from build123d import *

# Parameters (mm, degrees)
F0_W     = 38.1
F0_H     = 38.1
F0_R     = 6.35
F0_R_2   = 3.175
F1_DEPTH = 25.4
F2_W     = 21.117794
F2_H     = 7.199542
F2_W_2   = 19.090971
F3_DEPTH = 38.101


with BuildPart() as f1:
    # F0 (on Top) → F1 (new body)
    with BuildSketch(Plane.XY):
        with Locations((19.05, 19.05)):
            Rectangle(F0_W, F0_H)
        with Locations((19.05, 19.05)):
            Circle(F0_R, mode=Mode.SUBTRACT)
        with BuildLine():
            Line((69.85, 38.1), (38.1, 38.1))
            Line((38.1, 38.1), (38.1, 0))
            Line((38.1, 0), (69.85, 0))
            ThreePointArc((69.85, 0), (88.9, 19.05), (69.85, 38.1))
        make_face()
        with Locations((54.437503, 8.829627)):
            Circle(F0_R_2, mode=Mode.SUBTRACT)
        with Locations((69.85, 8.829627)):
            Circle(F0_R_2, mode=Mode.SUBTRACT)
        with Locations((54.437503, 29.22605)):
            Circle(F0_R_2, mode=Mode.SUBTRACT)
        with Locations((69.85, 29.22605)):
            Circle(F0_R_2, mode=Mode.SUBTRACT)
    extrude(amount=F1_DEPTH)

    # F2 (on face) → F3 (cut, through all)
    with BuildSketch(Plane.XZ):
        with Locations((59.291103, 21.800229)):
            Rectangle(F2_W, F2_H)
        with Locations((79.395485, 21.800229)):
            Rectangle(F2_W_2, F2_H)
        with Locations((59.291103, 3.599771)):
            Rectangle(F2_W, F2_H)
        with Locations((79.395485, 3.599771)):
            Rectangle(F2_W_2, F2_H)
    extrude(amount=-F3_DEPTH, mode=Mode.SUBTRACT)


solid = f1.part
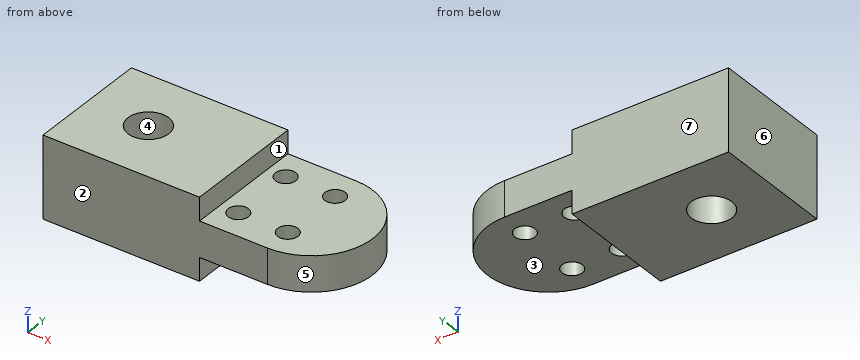
Input: part model. Units: mm. Frame: model coordinates. Face numbers are marked on the shaded views. A direction names the side the tool comes from. Round coordinates to 2 decimals unless told otherwise and drop trailing zeros. Order: outer loops, then holes, each group sorted by start corner. A loop starts at its lowest first (then second) coordinate and runs counter-clockwise, first axis right, second up.
1. Material intervals for line 1 (Y direction, x = 69.85, z = 15); line 2 (X direction, y = 31.5, z = 10); line 3 (Y direction, x = 19.05, z = 6.5), sorted ascending.
The answers:
line 1: y = 0 to 5.65, 12 to 26.05, 32.4 to 38.1
line 2: x = 0 to 52.22, 56.65 to 67.63, 72.07 to 84.27
line 3: y = 0 to 12.7, 25.4 to 38.1
2. Cut plane C-C, the plane y = 27. Output: boundary loops of the cut face in (x, z), then the cut area to 3 significant figures.
The answers:
outline: (0, 0) - (48.73, 0) - (48.73, 7.2) - (52.17, 7.2) - (52.17, 18.2) - (48.73, 18.2) - (48.73, 25.4) - (0, 25.4) - close; (56.7, 7.2) - (67.59, 7.2) - (67.59, 18.2) - (56.7, 18.2) - close; (72.11, 7.2) - (87.16, 7.2) - (87.16, 18.2) - (72.11, 18.2) - close
area: 1,560 mm2
3. Cut plane B-B, the plane y = 19.05. Output: boundary loops of the cut face in (x, z).
The answers:
outline: (0, 0) - (12.7, 0) - (12.7, 25.4) - (0, 25.4) - close; (25.4, 0) - (48.73, 0) - (48.73, 7.2) - (88.9, 7.2) - (88.9, 18.2) - (48.73, 18.2) - (48.73, 25.4) - (25.4, 25.4) - close
4. Mould query, pull axis X, two halves, no side actions, for the marked faces 4, 5, 6 and 7. Classes: released by +X, released by -X, zero draft, split by the parting line, or undercut.
The answers:
face 4: undercut
face 5: released by +X
face 6: released by -X
face 7: zero draft
5. Cut plane A-A, the plane x = 19.05. Output: boundary loops of the cut face in (y, z).
The answers:
outline: (0, 0) - (12.7, 0) - (12.7, 25.4) - (0, 25.4) - close; (25.4, 0) - (38.1, 0) - (38.1, 25.4) - (25.4, 25.4) - close
6. Cut plane D-D, the plane z = 20. Output: boundary loops of the cut face in (x, y).
The answers:
outline: (0, 0) - (48.73, 0) - (48.73, 38.1) - (0, 38.1) - close; hole circle Ø12.7 at (19.05, 19.05)
7. Set-up query: the marked faces 1, 2 and 3. Return all of +Z, -Z, +X, -X, +Y, -Y with unobstructed straight access to the full face (end or side cutting, diameter ignored); none if empty.
The answers:
face 1: +Z, +X, +Y, -Y
face 2: +Z, -Z, +X, -X, -Y
face 3: -Z, +X, +Y, -Y
8. Pin query (flat end, axial travel): P1, Ø3, axis at y = 9.5, z = 8.5, coming from the +X side; P2, Ø7.5, axis at x = 54.44, y = 8.83, coming from the +Z side; P3, Ø4, axis at x = 69.85, y = 29.23, coming from the -Z side; P4, Ø5, axis at x = 78.5, y = 21.5, coming from the -Z side. Return the tip coordinate at first contact, or that it passes through.
The answers:
P1: stops at x = 87.12
P2: stops at z = 18.2
P3: passes through
P4: stops at z = 7.2
